For this review, take the finished solid that the model builds, in its own axes (mm). A direction names the side the tool comes from. Coordinates: 2 decimals unless noted, no trailing zeros. Order: outer loops, then holes, each group sorted by start corner. A loop starts at its lowest first (then second) coordinate and runs counter-clockwise, first axis right, second up.
from build123d import *

# Parameters (mm, degrees)
F3_DEPTH = 330.2
F4_D     = 12.7
F4_DEPTH = 19.051
F5_D     = 12.7
F6_D     = 9.525
F6_DEPTH = 19.051
F2_D     = 9.525


with BuildPart() as f3:
    # F0 (on Front) → F3 (new body)
    with BuildSketch(Plane.XZ):
        with BuildLine():
            Line((-15.875, -19.05), (15.875, -19.05))
            ThreePointArc((15.875, -19.05), (18.1200640303, -18.1200640303), (19.05, -15.875))
            Line((19.05, -15.875), (19.05, 15.875))
            ThreePointArc((19.05, 15.875), (18.1200640303, 18.1200640303), (15.875, 19.05))
            Line((15.875, 19.05), (-15.875, 19.05))
            ThreePointArc((-15.875, 19.05), (-18.1200640303, 18.1200640303), (-19.05, 15.875))
            Line((-19.05, 15.875), (-19.05, -15.875))
            ThreePointArc((-19.05, -15.875), (-18.1200640303, -18.1200640303), (-15.875, -19.05))
        make_face()
        with BuildLine():
            ThreePointArc((14.2875, -11.1125), (13.3575640303, -13.3575640303), (11.1125, -14.2875))
            Line((11.1125, -14.2875), (-11.1125, -14.2875))
            ThreePointArc((-11.1125, -14.2875), (-13.3575640303, -13.3575640303), (-14.2875, -11.1125))
            Line((-14.2875, -11.1125), (-14.2875, 11.1125))
            ThreePointArc((-14.2875, 11.1125), (-13.3575640303, 13.3575640303), (-11.1125, 14.2875))
            Line((-11.1125, 14.2875), (11.1125, 14.2875))
            ThreePointArc((11.1125, 14.2875), (13.3575640303, 13.3575640303), (14.2875, 11.1125))
            Line((14.2875, 11.1125), (14.2875, -11.1125))
        make_face(mode=Mode.SUBTRACT)
    extrude(amount=F3_DEPTH)

    # F4 (through all, one way)
    with BuildSketch(Plane.XY):
        with Locations((0, -19.05)):
            Circle(F4_D / 2)
    extrude(amount=-F4_DEPTH, mode=Mode.SUBTRACT)

    # F5 (through all)
    with Locations(Plane(origin=(0, 0, 0), x_dir=(1, 0, 0), z_dir=(0, 0, -1))):
        with Locations((0, 19.05)):
            Hole(F5_D / 2)

    # F6 (through all, one way)
    with BuildSketch(Plane.XY):
        with Locations((0, -50.8)):
            Circle(F6_D / 2)
    extrude(amount=-F6_DEPTH, mode=Mode.SUBTRACT)

    # F2 (through all)
    with Locations(Plane(origin=(0, 0, 0), x_dir=(1, 0, 0), z_dir=(0, 0, -1))):
        with Locations((0, 50.8)):
            Hole(F2_D / 2)


solid = f3.part
1. Take a section at A-A, the plane z = -1. Give the boundary of the cut face in (x, y), plus the area to 3 significant figures.
Answer below:
outline: (-19.05, -330.2) - (-14.29, -330.2) - (-14.29, 0) - (-19.05, 0) - close; (14.29, -330.2) - (19.05, -330.2) - (19.05, 0) - (14.29, 0) - close
area: 3,150 mm2
2. To check wall thickness, follow L1, parallel to Y at x = 0, z = -16; L2, parallel to Z at x = 4.5, y = -81. State the ranges of each line that lie inside material, in increasing order.
Answer below:
L1: y = -330.2 to -55.56, -46.04 to -25.4, -12.7 to 0
L2: z = -19.05 to -14.29, 14.29 to 19.05
3. Take a section at B-B, the plane x = 0. Give the boundary of the cut face in (y, z).
Answer below:
outline: (-330.2, -19.05) - (-55.56, -19.05) - (-55.56, -14.29) - (-330.2, -14.29) - close; (-330.2, 14.29) - (-55.56, 14.29) - (-55.56, 19.05) - (-330.2, 19.05) - close; (-46.04, -19.05) - (-25.4, -19.05) - (-25.4, -14.29) - (-46.04, -14.29) - close; (-46.04, 14.29) - (-25.4, 14.29) - (-25.4, 19.05) - (-46.04, 19.05) - close; (-12.7, -19.05) - (0, -19.05) - (0, -14.29) - (-12.7, -14.29) - close; (-12.7, 14.29) - (0, 14.29) - (0, 19.05) - (-12.7, 19.05) - close
4. The part is to be moulded in two halves that separate along Y. For faces 3 (the face through (0, 0, -17)), 4 (the face through (0, -330.2, -17)), 5 (the face through (3.51, -54.02, 16.7)), say which applies: +Y half, -Y half, draft (parallel to the pull), parting line (faces both ways), or undercut.
Answer below:
face 3: +Y half
face 4: -Y half
face 5: undercut
5. Machinability: for faces 1 (the face through (-3.414, -24.404, 16.702)), 2 (the face through (-14.288, -163, 0)), which of the approach directions +Z, -Z, +X, -X, +Y, -Y give a long, thin tool a straight path to every point of the face, cutting with its end or side? Answer none if there is none.
Answer below:
face 1: +Z, -Z
face 2: +Y, -Y
